Check sheet for the modelled part. Datum: model origin and axes. Units: mm. Give positions to 0.01 mm unless a question says otherwise; leave off trailing zeros. Order: outer loops, then holes, each group sorted by start corner. A loop starts at its lowest first (then second) coordinate and runs counter-clockwise, first axis right, second up. Notation, with made-up numbers: (20, -22.5) - (58, -22.5) arc R32 cw to (58, 15.5) - close; hole circle Ø4 at (41, -5.75). An arc over 180 degrees is marked (long way). Answer in a Markdown table with one row per item.
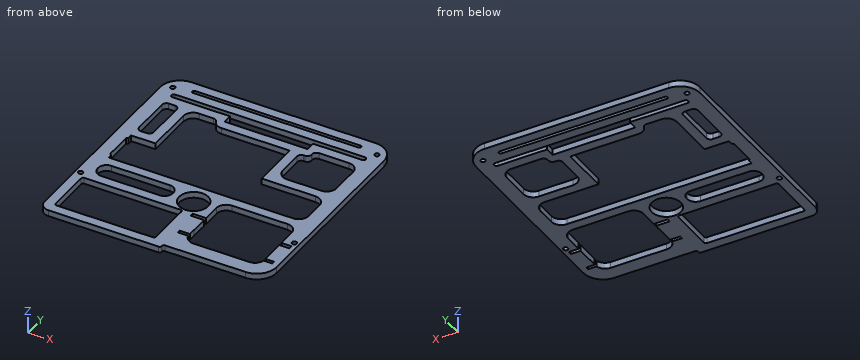
from build123d import *

# Parameters (mm, degrees)
SKETCH1_W           = 57.8674
SKETCH1_H           = 58.2902
SKETCH1_W_2         = 50.2474
SKETCH1_H_2         = 50.6702
BOSS_EXTRUDE1_DEPTH = 1.5875
SKETCH2_W           = 50.2474
SKETCH2_H           = 2.54
SKETCH2_H_2         = 2.1717
BOSS_EXTRUDE2_DEPTH = 1.5875
BOSS_EXTRUDE3_DEPTH = 1.5875
SKETCH4_W           = 11.3284
SKETCH4_H           = 17.169
BOSS_EXTRUDE4_DEPTH = 1.5875
SKETCH5_R           = 3.7592
SKETCH5_W           = 25.9588
SKETCH5_H           = 12.4587
CUT_EXTRUDE1_DEPTH  = 1.5875
SKETCH8_W           = 19.4595
SKETCH8_H           = 2.54
BOSS_EXTRUDE5_DEPTH = 1.5875
FILLET1_R           = 5.08
FILLET2_START       = -1
FILLET2_DEPTH       = 4
FILLET2_2_DEPTH     = 1.5875
FILLET3_R           = 1.0922
FILLET4_R           = 0.5842
FILLET8_R           = 2.159
SKETCH6_R           = 0.6096
CUT_EXTRUDE2_DEPTH  = 1.5875
SKETCH7_W           = 24.384
SKETCH7_H           = 0.8128
SKETCH7_W_2         = 19.05
SKETCH7_H_2         = 1.8796
SKETCH7_W_3         = 25.5778
SKETCH7_H_3         = 0.9144
CUT_EXTRUDE3_DEPTH  = 1.5875
FILLET6_R           = 0.508
SKETCH9_W           = 43.6434
SKETCH9_H           = 0.9017
CUT_EXTRUDE4_DEPTH  = 1.5875
FILLET7_R           = 0.4318
FILLET9_R           = 2.54
SKETCH10_W          = 31.4737
SKETCH10_H          = 1.143
BOSS_EXTRUDE6_DEPTH = 1.5875
FILLET10_R          = 2.54
FILLET11_R          = 0.508


with BuildPart() as part:
    # Sketch1 → Boss-Extrude1 (new body)
    with BuildSketch(Plane.XY):
        with Locations((42.165860751, 32.260946044)):
            Rectangle(SKETCH1_W, SKETCH1_H)
        with Locations((42.165860751, 32.260946044)):
            Rectangle(SKETCH1_W_2, SKETCH1_H_2, mode=Mode.SUBTRACT)
    extrude(amount=BOSS_EXTRUDE1_DEPTH)

    # Sketch2 → Boss-Extrude2 (add)
    with BuildSketch(Plane(origin=(0, 0, 0), x_dir=(-1, 0, 0), z_dir=(0, 0, -1))):
        with Locations((-42.165860751, 25.364846044)):
            Rectangle(SKETCH2_W, SKETCH2_H)
        Polygon((-67.289560751, 54.192446044), (-53.964160751, 54.192446044), (-53.964160751, 51.766746044), (-32.526560751, 51.766746044), (-32.526560751, 54.192446044), (-17.042160751, 54.192446044), (-17.042160751, 51.652446044), (-30.621560751, 51.652446044), (-30.621560751, 49.226746044), (-55.869160751, 49.226746044), (-55.869160751, 51.652446044), (-67.289560751, 51.652446044), align=None)
        with Locations((-42.165860751, 56.510196044)):
            Rectangle(SKETCH2_W, SKETCH2_H_2)
    extrude(amount=-BOSS_EXTRUDE2_DEPTH)

    # Sketch3 → Boss-Extrude3 (add)
    with BuildSketch(Plane(origin=(0, 0, 0), x_dir=(-1, 0, 0), z_dir=(0, 0, -1))):
        Polygon((-57.820560751, 36.634846044), (-50.820560751, 36.634846044), (-50.820560751, 28.408046044), (-50.820560751, 49.226746044), (-53.360560751, 49.226746044), (-53.360560751, 39.174846044), (-67.289560751, 39.174846044), (-67.289560751, 36.634846044), align=None)
        Polygon((-23.370560751, 36.634846044), (-20.120560751, 36.634846044), (-17.042160751, 36.634846044), (-17.042160751, 39.174846044), (-20.830560751, 39.174846044), (-20.830560751, 51.652446044), (-23.370560751, 51.652446044), align=None)
    extrude(amount=-BOSS_EXTRUDE3_DEPTH)

    # Sketch4 → Boss-Extrude4 (add)
    with BuildSketch(Plane(origin=(0, 0, 0), x_dir=(-1, 0, 0), z_dir=(0, 0, -1))):
        with Locations((-42.165860751, 15.510346044)):
            Rectangle(SKETCH4_W, SKETCH4_H)
    extrude(amount=-BOSS_EXTRUDE4_DEPTH)

    # Sketch5 → Cut-Extrude1 (cut)
    with BuildSketch(Plane(origin=(0, 0, 0), x_dir=(-1, 0, 0), z_dir=(0, 0, -1))):
        with Locations((-42.165860751, 21.224646044)):
            Circle(SKETCH5_R)
        with Locations((-28.783160751, 10.742196044)):
            Rectangle(SKETCH5_W, SKETCH5_H)
    extrude(amount=-CUT_EXTRUDE1_DEPTH, mode=Mode.SUBTRACT)

    # Sketch8 → Boss-Extrude5 (add)
    with BuildSketch(Plane(origin=(0, 0, 0), x_dir=(-1, 0, 0), z_dir=(0, 0, -1))):
        with Locations((-26.771910751, 18.241546044)):
            Rectangle(SKETCH8_W, SKETCH8_H)
    extrude(amount=-BOSS_EXTRUDE5_DEPTH)

    # Fillet1
    fillet1_edges = [part.edges().sort_by_distance(p)[0] for p in [
        (13.232160751, 61.406046044, 0.79375),
        (71.099560751, 61.406046044, 0.79375),
        (71.099560751, 3.115846044, 0.79375),
    ]]
    fillet(fillet1_edges, radius=FILLET1_R)

    # Fillet2: read off the stored shape, not the designer's step
    # Fillet2 outline → Fillet2 (cut)
    with BuildSketch(Plane.XY.offset(FILLET2_START)):
        with BuildLine():
            ThreePointArc((33.158987698, 49.226746044), (31.403812778, 49.930728342), (30.621560751, 51.652446044))
            Line((30.621560751, 51.652446044), (30.621560751, 49.226746044))
            Line((30.621560751, 49.226746044), (33.158987698, 49.226746044))
        make_face()
    extrude(amount=FILLET2_DEPTH, mode=Mode.SUBTRACT)

    # Fillet2 2 outline → Fillet2 2 (add)
    with BuildSketch(Plane.XY):
        with BuildLine():
            Line((67.289560751, 36.634846044), (64.749560751, 36.634846044))
            ThreePointArc((64.749560751, 36.634846044), (66.545611975, 35.890897268), (67.289560751, 34.094846044))
            Line((67.289560751, 34.094846044), (67.289560751, 36.634846044))
        make_face()
        with BuildLine():
            Line((67.289560751, 26.634846044), (67.289560751, 29.174846044))
            ThreePointArc((67.289560751, 29.174846044), (66.545611975, 27.37879482), (64.749560751, 26.634846044))
            Line((64.749560751, 26.634846044), (67.289560751, 26.634846044))
        make_face()
        with BuildLine():
            ThreePointArc((23.370560751, 49.112446044), (24.114509527, 50.908497268), (25.910560751, 51.652446044))
            Line((25.910560751, 51.652446044), (23.370560751, 51.652446044))
            Line((23.370560751, 51.652446044), (23.370560751, 49.112446044))
        make_face()
        with BuildLine():
            ThreePointArc((64.749560751, 51.652446044), (66.545611975, 50.908497268), (67.289560751, 49.112446044))
            Line((67.289560751, 49.112446044), (67.289560751, 51.652446044))
            Line((67.289560751, 51.652446044), (64.749560751, 51.652446044))
        make_face()
        with BuildLine():
            Line((53.360560751, 39.174846044), (55.900560751, 39.174846044))
            ThreePointArc((55.900560751, 39.174846044), (54.104509527, 39.91879482), (53.360560751, 41.714846044))
            Line((53.360560751, 41.714846044), (53.360560751, 39.174846044))
        make_face()
        with BuildLine():
            Line((67.289560751, 39.174846044), (67.289560751, 41.714846044))
            ThreePointArc((67.289560751, 41.714846044), (66.545611975, 39.91879482), (64.749560751, 39.174846044))
            Line((64.749560751, 39.174846044), (67.289560751, 39.174846044))
        make_face()
    extrude(amount=FILLET2_2_DEPTH)

    # Fillet3
    fillet3_edges = [part.edges().sort_by_distance(p)[0] for p in [
        (20.830560751, 51.652446044, 0.79375),
        (20.830560751, 39.174846044, 0.79375),
        (17.042160751, 39.174846044, 0.79375),
        (17.042160751, 51.652446044, 0.79375),
        (30.621560751, 51.652446044, 0.79375),
        (55.869160751, 49.226746044, 0.79375),
        (55.869160751, 51.652446044, 0.79375),
        (53.360560751, 49.226746044, 0.79375),
    ]]
    fillet(fillet3_edges, radius=FILLET3_R)

    # Fillet4
    fillet4_edges = [part.edges().sort_by_distance(p)[0] for p in [
        (17.042160751, 54.192446044, 0.79375),
        (67.289560751, 54.192446044, 0.79375),
        (67.289560751, 55.424346044, 0.79375),
        (17.042160751, 55.424346044, 0.79375),
    ]]
    fillet(fillet4_edges, radius=FILLET4_R)

    # Fillet8
    fillet8_edges = [part.edges().sort_by_distance(p)[0] for p in [
        (36.501660751, 24.094846044, 0.79375),
        (36.501660751, 19.511546044, 0.79375),
        (17.042160751, 19.511546044, 0.79375),
        (17.042160751, 24.094846044, 0.79375),
    ]]
    fillet(fillet8_edges, radius=FILLET8_R)

    # Sketch6 → Cut-Extrude2 (cut)
    with BuildSketch(Plane(origin=(0, 0, 0), x_dir=(-1, 0, 0), z_dir=(0, 0, -1))):
        with Locations((-68.559560751, 57.596046044)):
            Circle(SKETCH6_R)
        with Locations((-14.527560751, 18.430646044)):
            Circle(SKETCH6_R)
        with Locations((-69.804160751, 18.430646044)):
            Circle(SKETCH6_R)
        with Locations((-15.772160751, 57.596046044)):
            Circle(SKETCH6_R)
        Polygon((-16.620560751, 28.134846044), (-18.120560751, 26.634846044), (-18.120560751, 36.634846044), (-16.620560751, 35.134846044), align=None)
    extrude(amount=-CUT_EXTRUDE2_DEPTH, mode=Mode.SUBTRACT)

    # Sketch7 → Cut-Extrude3 (cut)
    with BuildSketch(Plane(origin=(0, 0, 0), x_dir=(-1, 0, 0), z_dir=(0, 0, -1))):
        with Locations((-57.328560751, 9.368745978)):
            Rectangle(SKETCH7_W, SKETCH7_H)
        with Locations((-57.328560751, 10.714945978)):
            Rectangle(SKETCH7_W_2, SKETCH7_H_2)
        with Locations((-57.091460751, 16.514346044)):
            Rectangle(SKETCH7_W_3, SKETCH7_H_3)
    extrude(amount=-CUT_EXTRUDE3_DEPTH, mode=Mode.SUBTRACT)

    # Fillet6
    fillet6_edges = [part.edges().sort_by_distance(p)[0] for p in [
        (15.803760751, 16.971546044, 0.79375),
        (15.803760751, 4.512846044, 0.79375),
        (41.762560751, 4.512846044, 0.79375),
        (41.762560751, 16.971546044, 0.79375),
    ]]
    fillet(fillet6_edges, radius=FILLET6_R)

    # Sketch9 → Cut-Extrude4 (cut)
    with BuildSketch(Plane.XY.offset(1.5875)):
        with Locations((42.165860751, 58.415196044)):
            Rectangle(SKETCH9_W, SKETCH9_H)
    extrude(amount=-CUT_EXTRUDE4_DEPTH, mode=Mode.SUBTRACT)

    # Fillet7
    fillet7_edges = [part.edges().sort_by_distance(p)[0] for p in [
        (63.987560751, 57.964346044, 0.79375),
        (63.987560751, 58.866046044, 0.79375),
        (20.344160751, 58.866046044, 0.79375),
        (20.344160751, 57.964346044, 0.79375),
    ]]
    fillet(fillet7_edges, radius=FILLET7_R)

    # Fillet9
    # the kernel refuses this fillet: 2.54 mm, written as the material it adds along each edge
    with BuildSketch(Plane(origin=(47.830060751, 6.925846044, 0), x_dir=(1, 0, 0), z_dir=(0, 0, 1))) as fillet9_piece_1:
        with BuildLine():
            CenterArc((2.489595888, 2.54), FILLET9_R, 191.433378163, 78.566621837)
            Line((0, 2.036499934), (-0.049791918, 2.026429933))
            ThreePointArc((-0.049791918, 2.026429933), (-0.0508, 1.018249967), (-0.0508, 0))
            Line((-0.0508, 0), (0, -0.0508))
            Line((0, -0.0508), (2.489595888, -0.0508))
            Line((2.489595888, -0.0508), (2.489595888, 0))
        make_face()
    extrude(amount=1.5875)
    with BuildSketch(Plane(origin=(47.830060751, 24.094846044, 0), x_dir=(1, 0, 0), z_dir=(0, 0, 1)), Plane(origin=(67.289560751, 24.094846044, 0), x_dir=(0, -1, 0), z_dir=(0, 0, 1))) as fillet9_piece_2:
        with BuildLine():
            CenterArc((FILLET9_R, -FILLET9_R), FILLET9_R, 90, 90)
            Line((0, -FILLET9_R), (-FILLET9_R * 0.02, -FILLET9_R))
            Line((-FILLET9_R * 0.02, -FILLET9_R), (-FILLET9_R * 0.02, FILLET9_R * 0.02))
            Line((-FILLET9_R * 0.02, FILLET9_R * 0.02), (FILLET9_R, FILLET9_R * 0.02))
            Line((FILLET9_R, FILLET9_R * 0.02), (FILLET9_R, 0))
        make_face()
    extrude(amount=1.5875)
    with BuildSketch(Plane(origin=(67.289560751, 6.925846044, 0), x_dir=(-1.3886374564076336e-12, 1.0, 0), z_dir=(0, 0, 1))) as fillet9_piece_3:
        with BuildLine():
            CenterArc((2.54, 2.489595888), FILLET9_R, 180, 78.566621837)
            Line((0, 2.489595888), (-0.0508, 2.489595888))
            Line((-0.0508, 2.489595888), (-0.0508, 0))
            Line((-0.0508, 0), (0, -0.0508))
            ThreePointArc((0, -0.0508), (1.018249967, -0.0508), (2.026429933, -0.049791918))
            Line((2.026429933, -0.049791918), (2.036499934, 0))
        make_face()
    extrude(amount=1.5875)

    # Sketch10 → Boss-Extrude6 (add)
    with BuildSketch(Plane.XY.offset(1.5875)):
        with Locations((28.969010751, 2.544346044)):
            Rectangle(SKETCH10_W, SKETCH10_H)
    extrude(amount=-BOSS_EXTRUDE6_DEPTH)

    # Fillet10
    fillet10_edges = [part.edges().sort_by_distance(p)[0] for p in [
        (13.232160751, 1.972846044, 0.79375),
    ]]
    fillet(fillet10_edges, radius=FILLET10_R)

    # Fillet11
    fillet11_edges = [part.edges().sort_by_distance(p)[0] for p in [
        (44.705860751, 1.972846044, 0.79375),
        (44.705860751, 3.115846044, 0.79375),
    ]]
    fillet(fillet11_edges, radius=FILLET11_R)


solid = part.part
(1) Cross-section at D-D, the plane z = 0.7. Give the number of separate pieces and of enclosed holes in the cut face, then the cut area to 3 significant figures.
Geometry says:
| item | result |
|---|---|
| separate pieces | 1 |
| enclosed holes | 13 |
| area | 1,370 mm² |
(2) Cross-section at B-B, the plane x = 22. Record the cut outline in (y, z).
Geometry says:
| item | result |
|---|---|
| outline | (1.97, 0) - (4.51, 0) - (4.51, 1.59) - (1.97, 1.59) - close; (16.97, 0) - (19.51, 0) - (19.51, 1.59) - (16.97, 1.59) - close; (24.09, 0) - (26.63, 0) - (26.63, 1.59) - (24.09, 1.59) - close; (36.63, 0) - (54.19, 0) - (54.19, 1.59) - (36.63, 1.59) - close; (55.42, 0) - (57.96, 0) - (57.96, 1.59) - (55.42, 1.59) - close; (58.87, 0) - (61.41, 0) - (61.41, 1.59) - (58.87, 1.59) - close |
(3) Cross-section at A-A, the plane y = 15. Record the cut outline in (x, z), then the cut area to 3 significant figures.
Geometry says:
| item | result |
|---|---|
| outline | (13.23, 0) - (15.8, 0) - (15.8, 1.59) - (13.23, 1.59) - close; (41.76, 0) - (47.83, 0) - (47.83, 1.59) - (41.76, 1.59) - close; (67.29, 0) - (71.1, 0) - (71.1, 1.59) - (67.29, 1.59) - close |
| area | 19.8 mm² |
(4) Gauge pin test, flat ends, axial feed: P1, Ø0.5, axis at x = 60, z = 1, coming from the -Y side; P2, Ø3, axis at x = 32, y = 47, coming from the -Z side. Record the tip position at first contact, or that the pin passes through.
Geometry says:
| item | result |
|---|---|
| P1 | y = 3.12 |
| P2 | through |
(5) Thickness scan on L1, parallel to Y at x = 61, z = 0.9; L2, parallel to Y at x = 33.5, z = 1; L3, parallel to X at y = 48, z = 0.25. Record the ranges inside material, lowest first.
Geometry says:
| item | result |
|---|---|
| L1 | 3.12 to 6.93, 24.09 to 26.63, 36.63 to 39.17, 51.65 to 54.19, 55.42 to 57.96, 58.87 to 61.41 |
| L2 | 1.97 to 4.51, 16.97 to 19.51, 24.09 to 26.63, 49.23 to 51.77, 55.42 to 57.96, 58.87 to 61.41 |
| L3 | 13.23 to 17.04, 20.83 to 23.37, 50.82 to 53.36, 67.29 to 71.1 |
(6) Cross-section at C-C, the plane y = 23. Record the cut outline in (x, z).
Geometry says:
| item | result |
|---|---|
| outline | (13.23, 0) - (17.32, 0) - (17.32, 1.59) - (13.23, 1.59) - close; (36.22, 0) - (38.85, 0) - (38.85, 1.59) - (36.22, 1.59) - close; (45.48, 0) - (48.28, 0) - (48.28, 1.59) - (45.48, 1.59) - close; (66.84, 0) - (71.1, 0) - (71.1, 1.59) - (66.84, 1.59) - close |
